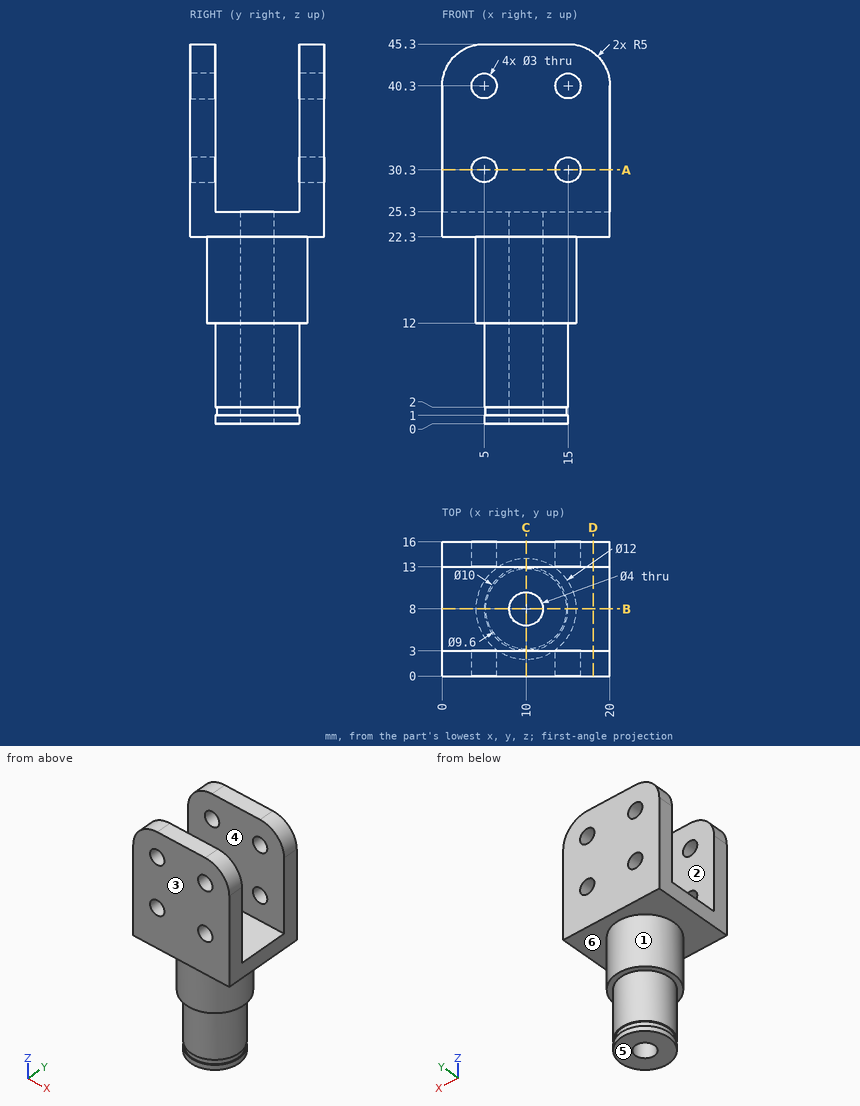
The drawing under review shows one solid part. Ordinate dimensions are in mm from its lowest x, y, z. A direction names the side the tool comes from. Give positions to 0.01 mm unless a question says otherwise; leave off trailing zeros. Write each loop counter-clockwise with the first axis right and the second up, starting at its lowest first coordinate (ties: lowest second). Pieces come first, ordered by that corner, then holes.
1. Add section A-A, the plane z = 30.3. Write out the cut boundary in (x, y).
2. Add section B-B, the plane y = 8. Write out the cut boundary in (x, z), plus the area to 3 significant figures.
3. For P1, Ø3, axis at x = 17.5, y = 4, coming from the +Z side; P2, Ø2.5, axis at x = 15, z = 30.3, coming from the +Y side; P3, Ø5, axis at y = 8, z = 15.5, coming from the -X side; P4, Ø8, axis at y = 14, z = 13, coming from the +X side, all flat-tipped, find the tip position at first contact; note any pin that passes through.
4. Draft analysis for pull direction Y (two halves, no side actions). For the marked faces 1, 2 and 3, state which applies: +Y half, -Y half, draft (parallel to the pull), parting line (faces both ways), or undercut.
5. Tool access review of the marked faces 4, 5 and 6: name each direction out of +Z, -Z, +X, -X, +Y, -Y from which nothing blocks a thin tool from reaching the whole face with its end or side.
6. Wall thickness on L1, parallel to X at y = 1.2, z = 30.3; L2, parallel to Y at x = 11.75, z = 38.5; L3, parallel to Z at x = 5.5, y = 11.75: over which ranges is each line inside the solid? List them lowest first.
7. Add section D-D, the plane x = 18. Write out the cut boundary in (y, z), plus the area to 3 significant figures.
8. Add section C-C, the plane x = 10. Write out the cut boundary in (y, z).
Worked answers:
1. outline: (0, 0) - (3.5, 0) - (3.5, 3) - (0, 3) - close; (0, 13) - (3.5, 13) - (3.5, 16) - (0, 16) - close; (6.5, 0) - (13.5, 0) - (13.5, 3) - (6.5, 3) - close; (6.5, 13) - (13.5, 13) - (13.5, 16) - (6.5, 16) - close; (16.5, 0) - (20, 0) - (20, 3) - (16.5, 3) - close; (16.5, 13) - (20, 13) - (20, 16) - (16.5, 16) - close
2. outline: (0, 22.3) - (4, 22.3) - (4, 12) - (5, 12) - (5, 2) - (5.2, 2) - (5.2, 1) - (5, 1) - (5, 0) - (8, 0) - (8, 25.3) - (0, 25.3) - close; (12, 0) - (15, 0) - (15, 1) - (14.8, 1) - (14.8, 2) - (15, 2) - (15, 12) - (16, 12) - (16, 22.3) - (20, 22.3) - (20, 25.3) - (12, 25.3) - close
2. area: 202 mm2
3. P1: stops at z = 45.11
3. P2: passes through
3. P3: stops at x = 4
3. P4: stops at x = 15.66
4. face 1: parting line
4. face 2: undercut
4. face 3: -Y half
5. face 4: +Z, +X, -X
5. face 5: -Z, +X, -X, +Y, -Y
5. face 6: -Z
6. L1: x = 0 to 3.5, 6.5 to 13.5, 16.5 to 20
6. L2: y = 0 to 3, 13 to 16
6. L3: z = 12 to 25.3
7. outline: (0, 22.3) - (16, 22.3) - (16, 44.3) - (13, 44.3) - (13, 25.3) - (3, 25.3) - (3, 44.3) - (0, 44.3) - close
7. area: 162 mm2
8. outline: (0, 22.3) - (2, 22.3) - (2, 12) - (3, 12) - (3, 2) - (3.2, 2) - (3.2, 1) - (3, 1) - (3, 0) - (6, 0) - (6, 25.3) - (3, 25.3) - (3, 45.3) - (0, 45.3) - close; (10, 0) - (13, 0) - (13, 1) - (12.8, 1) - (12.8, 2) - (13, 2) - (13, 12) - (14, 12) - (14, 22.3) - (16, 22.3) - (16, 45.3) - (13, 45.3) - (13, 25.3) - (10, 25.3) - close
